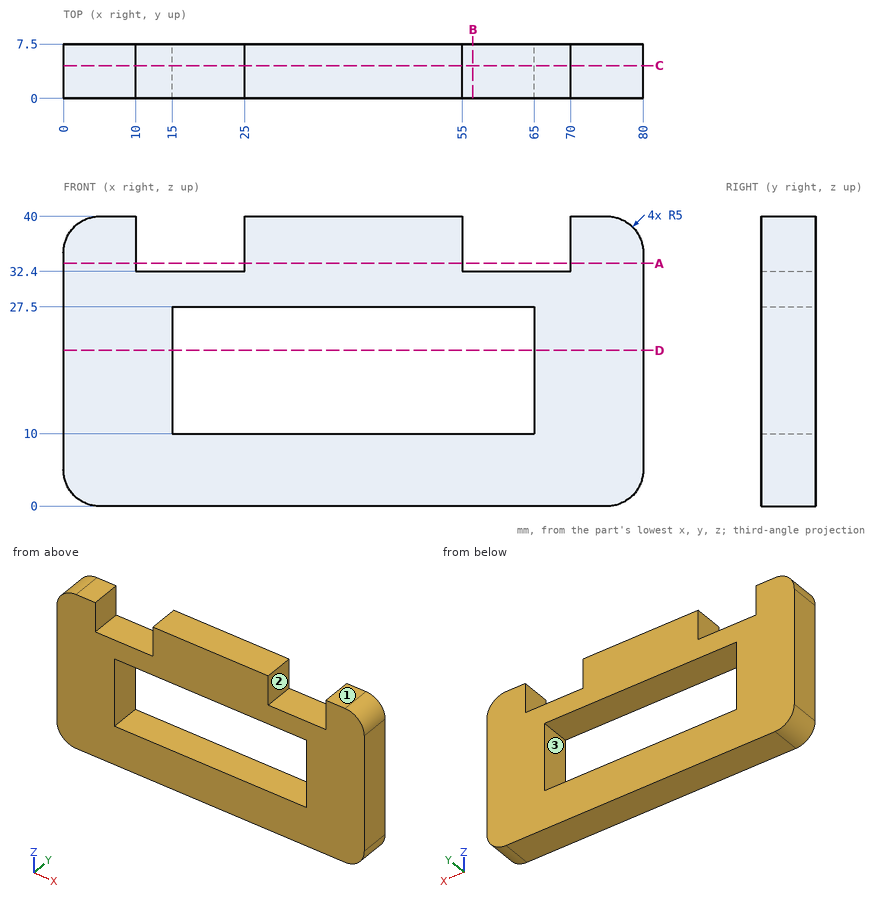
The figure shows three views and two pictorial views of one solid part (mm, origin at its lowest corner). Answer the questions. A direction names the side the tool comes from. Round coordinates to 2 decimals unless told otherwise and drop trailing zeros. Order: outer loops, then holes, each group sorted by start corner. A loop starts at its lowest first (then second) coordinate and runs counter-clockwise, first axis right, second up. Notation, with made-up numbers: M -1.5,-32 L 46.5,-32 A27 cw 46.5,-1 Z; hole C 40.25,82.25 d3. An arc over 180 degrees is marked long. Answer in a Markdown table with one row per item. Add a question column.
1) Which of the six approach directions +Z, -Z, +X, -X, +Y, -Y give full straight-line access (tool end or side, diameter ignored) to the marked faces 1, 2 and 3?
2) The part is cut by section A-A on z = 33.5. Determine the outline of the cut face in (x, y), plus the area to 3 significant figures.
3) The part is cut by section B-B on x = 56.5. Determine the outline of the cut face in (y, z), plus the area to 3 significant figures.
4) The part is cut by section C-C on y = 4.5. Determine the outline of the cut face in (x, z).
5) A flat-ended cylindrical pin translates along its axis: pin 1 Ø1.5 at (x, y) = (66.5, 2.5) entering from +Z. Find the tip coordinate at first contact, or state that the pin passes through.
6) Consider line 1 along Z through (x, y) = (62.5, 4); line 2 along Z through (x, y) = (32, 4.5); line 3 along X through (y, z) = (4.25, 12). Determine where each line is inside the solid, lowest interval first. Write a range as from..to.
7) The part is cut by section D-D on z = 21.5. Determine the outline of the cut face in (x, y), plus the area to 3 significant figures.
Findings below:
| question | item | result |
|---|---|---|
| 1 | face 1 | +Z, +X, -X, +Y, -Y |
| 1 | face 2 | +Z, +Y, -Y |
| 1 | face 3 | +Y, -Y |
| 2 | outline | M 0,0 L 10,0 L 10,7.5 L 0,7.5 Z; M 25,0 L 55,0 L 55,7.5 L 25,7.5 Z; M 70,0 L 80,0 L 80,7.5 L 70,7.5 Z |
| 2 | area | 375 mm² |
| 3 | outline | M 0,0 L 7.5,0 L 7.5,10 L 0,10 Z; M 0,27.5 L 7.5,27.5 L 7.5,32.4 L 0,32.4 Z |
| 3 | area | 112 mm² |
| 4 | outline | M 0,5 A5 ccw 5,0 L 75,0 A5 ccw 80,5 L 80,35 A5 ccw 75,40 L 70,40 L 70,32.4 L 55,32.4 L 55,40 L 25,40 L 25,32.4 L 10,32.4 L 10,40 L 5,40 A5 ccw 0,35 Z; hole M 15,10 L 65,10 L 65,27.5 L 15,27.5 Z |
| 5 | pin 1 | stops at z = 32.4 |
| 6 | line 1 | z = 0..10, 27.5..32.4 |
| 6 | line 2 | z = 0..10, 27.5..40 |
| 6 | line 3 | x = 0..15, 65..80 |
| 7 | outline | M 0,0 L 15,0 L 15,7.5 L 0,7.5 Z; M 65,0 L 80,0 L 80,7.5 L 65,7.5 Z |
| 7 | area | 225 mm² |
